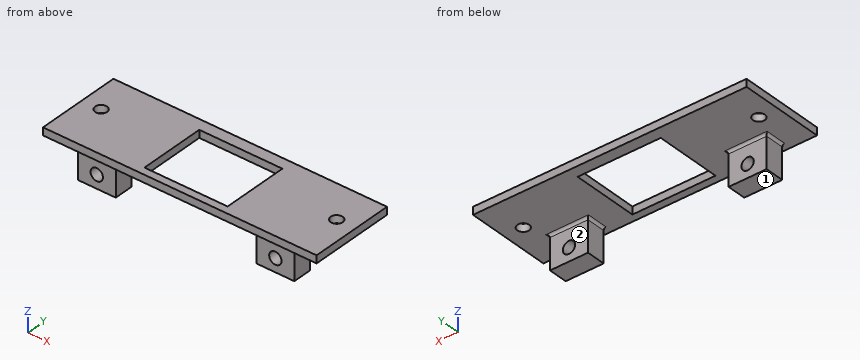
from build123d import *

# Parameters (mm, degrees)
SKETCH1_W               = 57.6
SKETCH1_H               = 18
SKETCH1_R               = 1.25
BOSS_EXTRUDE1_DEPTH     = 1.6
SKETCH7_W               = 8
SKETCH7_H               = 7
SKETCH7_R               = 1.3
BOSS_EXTRUDE3_DEPTH     = 4
BOSS_EXTRUDE3_2_DEPTH   = 4
CUT_EXTRUDE1_DEPTH      = 35.676216633
CUT_EXTRUDE1_DEPTH_BACK = 35.676216633
SKETCH8_W               = 17.5
SKETCH8_H               = 14
FILLET1_R               = 0.5


with BuildPart() as part:
    # Sketch1 → Boss-Extrude1 (new body)
    with BuildSketch(Plane.XY):
        with Locations((0, 9)):
            Rectangle(SKETCH1_W, SKETCH1_H)
        with Locations((-24.8, 10)):
            Circle(SKETCH1_R, mode=Mode.SUBTRACT)
        with Locations((24.8, 10)):
            Circle(SKETCH1_R, mode=Mode.SUBTRACT)
    extrude(amount=BOSS_EXTRUDE1_DEPTH)

    # Sketch8 → Cut-Extrude1 (cut, two sides: drawn at the far end of the back side and taken through both)
    with BuildSketch(Plane.XY.offset(-CUT_EXTRUDE1_DEPTH_BACK)):
        with Locations((0, 8.6)):
            Rectangle(SKETCH8_W, SKETCH8_H)
    extrude(amount=CUT_EXTRUDE1_DEPTH + CUT_EXTRUDE1_DEPTH_BACK, mode=Mode.SUBTRACT)


with BuildPart() as body_2:
    # Sketch7 → Boss-Extrude3 (new body)
    with BuildSketch(Plane(origin=(0, 1.6, 0), x_dir=(1, 0, 0), z_dir=(0, 1, 0))):
        with Locations((-18.8, 3.5)):
            Rectangle(SKETCH7_W, SKETCH7_H)
        with Locations(Location((-18.8, 4.2, 0), (0, 0, 270))):
            Circle(SKETCH7_R, mode=Mode.SUBTRACT)
    extrude(amount=BOSS_EXTRUDE3_DEPTH)


with BuildPart() as body_3:
    # Sketch7 → Boss-Extrude3 2 (new body)
    with BuildSketch(Plane(origin=(0, 1.6, 0), x_dir=(1, 0, 0), z_dir=(0, 1, 0))):
        with Locations((18.8, 3.5)):
            Rectangle(SKETCH7_W, SKETCH7_H)
        with Locations(Location((18.8, 4.2, 0), (0, 0, 270))):
            Circle(SKETCH7_R, mode=Mode.SUBTRACT)
    extrude(amount=BOSS_EXTRUDE3_2_DEPTH)


with BuildPart() as body_2_1:
    add(body_2.part)

    # Combine1: union part, body 3
    add(part.part)
    add(body_3.part)

    # Fillet1
    fillet1_edges = [body_2_1.edges().sort_by_distance(p)[0] for p in [
        (14.8, 3.6, 0),
        (18.8, 5.6, 0),
        (22.8, 3.6, 0),
        (-14.8, 3.6, 0),
        (-22.8, 3.6, 0),
        (-18.8, 5.6, 0),
    ]]
    fillet(fillet1_edges, radius=FILLET1_R)


solid = body_2_1.part
Design review of the part built by this model. Coordinates are the model's own, in mm. Face numbers are marked on the shaded views. A direction names the side the tool comes from. Coordinates: 2 decimals unless noted, no trailing zeros. Loops run counter-clockwise (first coordinate to the right, second up) from the corner with the lowest first, then second, coordinate; pieces in that order, holes last. Notation, with made-up numbers: (30.25, 75) -> (67.25, 75) arc R7 ccw to (67.25, 88) -> close; hole circle Ø8 at (-14.75, 83.5). An arc over 180 degrees is marked (long way). Use a Markdown table: item, result. Add a question column.
Item 1: We need section D-D, the plane y = 8. Write out the cut boundary in (x, z), and give its area (3 significant figures).
Item 2: Clearance check with flat-ended pins moving along their axes: P1, Ø1.5, axis at y = 8, z = -6, coming from the -X side; P2, Ø6, axis at x = -4.5, y = 2, coming from the -Z side; P3, Ø3, axis at y = 3, z = -3, coming from the -X side; P4, Ø4.5, axis at y = 4, z = -3.5, coming from the +X side. State where each tip first meets the part, or that it passes through.
Item 3: We need section B-B, the plane z = -4.2. Write out the cut boundary in (x, y), and give its area (3 significant figures).
Item 4: Wall thickness on L1, parallel to X at y = 3.2, z = -4.2; L2, parallel to Y at x = -24.8, z = 1.05; L3, parallel to X at y = 2.5, z = -1.75: over which ranges is each line inside the solid? List them lowest first. Write a range as from..to.
Item 5: We need section A-A, the plane x = -3.5. Write out the cut boundary in (y, z), and give its area (3 significant figures).
Item 6: We need section C-C, the plane y = 4. Write out the cut boundary in (x, z).
Item 7: Machinability: for the marked faces 1 and 2, which of the approach directions +Z, -Z, +X, -X, +Y, -Y give a long, thin tool a straight path to every point of the face, cutting with its end or side? Answer none if there is none.
Numbers:
| question | item | result |
|---|---|---|
| 1 | outline | (-28.8, 0) -> (-8.75, 0) -> (-8.75, 1.6) -> (-28.8, 1.6) -> close; (8.75, 0) -> (28.8, 0) -> (28.8, 1.6) -> (8.75, 1.6) -> close |
| 1 | area | 64.2 mm^2 |
| 2 | P1 | passes through |
| 2 | P2 | stops at z = 0 |
| 2 | P3 | stops at x = -22.8 |
| 2 | P4 | stops at x = 22.8 |
| 3 | outline | (-22.8, 1.6) -> (-20.1, 1.6) -> (-20.1, 5.6) -> (-22.8, 5.6) -> close; (-17.5, 1.6) -> (-14.8, 1.6) -> (-14.8, 5.6) -> (-17.5, 5.6) -> close; (14.8, 1.6) -> (17.5, 1.6) -> (17.5, 5.6) -> (14.8, 5.6) -> close; (20.1, 1.6) -> (22.8, 1.6) -> (22.8, 5.6) -> (20.1, 5.6) -> close |
| 3 | area | 43.2 mm^2 |
| 4 | L1 | x = -22.8..-20.1, -17.5..-14.8, 14.8..17.5, 20.1..22.8 |
| 4 | L2 | y = 0..8.75, 11.25..18 |
| 4 | L3 | x = -22.8..-14.8, 14.8..22.8 |
| 5 | outline | (0, 0) -> (1.6, 0) -> (1.6, 1.6) -> (0, 1.6) -> close; (15.6, 0) -> (18, 0) -> (18, 1.6) -> (15.6, 1.6) -> close |
| 5 | area | 6.40 mm^2 |
| 6 | outline | (-28.8, 0) -> (-23.3, 0) arc R0.5 cw to (-22.8, -0.5) -> (-22.8, -7) -> (-14.8, -7) -> (-14.8, -0.5) arc R0.5 cw to (-14.3, 0) -> (-8.75, 0) -> (-8.75, 1.6) -> (-28.8, 1.6) -> close; (8.75, 0) -> (14.3, 0) arc R0.5 cw to (14.8, -0.5) -> (14.8, -7) -> (22.8, -7) -> (22.8, -0.5) arc R0.5 cw to (23.3, 0) -> (28.8, 0) -> (28.8, 1.6) -> (8.75, 1.6) -> close; hole circle Ø2.6 at (-18.8, -4.2); hole circle Ø2.6 at (18.8, -4.2) |
| 7 | face 1 | -Z, +X, -X, +Y, -Y |
| 7 | face 2 | -Z, +X, -X, +Y |
